```python
from build123d import *

# Parameters (mm, degrees)
SALIENTE_EXTRUIR1_DEPTH = 1.5
CROQUIS2_R              = 1.6
CORTAR_EXTRUIR1_DEPTH   = 3
REDONDEO1_R             = 1
CROQUIS3_R              = 1.5
CORTAR_EXTRUIR2_DEPTH   = 5


with BuildPart() as part:
    # Croquis1 → Saliente-Extruir1 (new, symmetric)
    with BuildSketch(Plane.XY):
        with BuildLine():
            Line((-6, 51), (-6, -10))
            Line((-6, -10), (-3, -10))
            Line((-3, -10), (-3, -55))
            Line((-3, -55), (3, -55))
            Line((3, -55), (3, -10))
            Line((3, -10), (6, -10))
            Line((6, -10), (6, 51))
            ThreePointArc((6, 51), (4.828427125, 53.828427125), (2, 55))
            Line((2, 55), (-2, 55))
            ThreePointArc((-2, 55), (-4.828427125, 53.828427125), (-6, 51))
        make_face()
    extrude(amount=SALIENTE_EXTRUIR1_DEPTH, both=True)

    # Croquis2 → Cortar-Extruir1 (cut)
    with BuildSketch(Plane.XY.offset(1.5)):
        with Locations((0, 50)):
            Circle(CROQUIS2_R)
    extrude(amount=-CORTAR_EXTRUIR1_DEPTH, mode=Mode.SUBTRACT)

    # Redondeo1
    redondeo1_edges = [part.edges().sort_by_distance(p)[0] for p in [
        (3, -55, 0),
        (-3, -55, 0),
    ]]
    fillet(redondeo1_edges, radius=REDONDEO1_R)

    # Croquis3 → Cortar-Extruir2 (cut, symmetric)
    with BuildSketch(Plane.XY):
        Circle(CROQUIS3_R)
    extrude(amount=CORTAR_EXTRUIR2_DEPTH, both=True, mode=Mode.SUBTRACT)


solid = part.part
```
The listing builds one solid part. Answer for the finished solid, in the listing's coordinates (mm). A direction names the side the tool comes from. Round coordinates to 2 decimals unless told otherwise and drop trailing zeros. Order: outer loops, then holes, each group sorted by start corner. A loop starts at its lowest first (then second) coordinate and runs counter-clockwise, first axis right, second up. Notation, with made-up numbers: (82, -3) -> (128, -3) arc R23 cw to (128, 18) -> close; hole circle Ø5 at (6, 24.5). An arc over 180 degrees is marked (long way). Answer as CSV lines item,"result". Start each with the question number.
(1) A tool of negligible diameter and unlimited length cuts with its end or side. For faces 1 (the face through (-6, 21, 0)), 2 (the face through (4, -10, 0)), 3 (the face through (-3, -32, 0)), from which of +Z, -Z, +X, -X, +Y, -Y can it reach the whole face along a straight path? Write none if from no direction.
(2) For a pull along Y with two mould halves and no side action, classify faces 4 (the face through (4.859, 53.797, 0.021)), 5 (the face through (6, 20, 0)), 6 (the face through (-1.5, 0.07, 0.02)) as +Y half, -Y half, draft (parallel to the pull), parting line (faces both ways), or undercut.
(3) Flat-ended cylindrical pins translate along their axes: pin 1 Ø4 at (x, y) = (0, 50) entering from +Z; pin 2 Ø0.9 at (y, z) = (-39.5, -0.5) entering from -X. Find the tip coordinate at first contact, or state that the pin passes through.
(4) The part is cut by section B-B (y = 0). Determine the outline of the cut face in (x, z).
(5) The part is cut by section A-A (x = 0). Determine the outline of the cut face in (y, z).
(6) The part is cut by section D-D (y = -13.5). Determine the outline of the cut face in (x, z), then the cut area to 3 significant figures.
(7) Find the intervals of material crossed by probe 1 along Y at (x, z) = (0, 0.15); probe 2 along Y at (x, z) = (1.25, 0.3); probe 3 along X at (y, z) = (-39, -1), in increasing order. Write a range as from..to.
(8) The part is cut by section C-C (y = 50). Determine the outline of the cut face in (x, z), then the cut area to 3 significant figures.
Evaluation:
1,face 1,"+Z, -Z, -X, +Y, -Y"
1,face 2,"+Z, -Z, +X, -Y"
1,face 3,"+Z, -Z, -X, -Y"
2,face 4,"+Y half"
2,face 5,"draft"
2,face 6,"undercut"
3,pin 1,"z = 1.5"
3,pin 2,"x = -3"
4,outline,"(-6, -1.5) -> (-1.5, -1.5) -> (-1.5, 1.5) -> (-6, 1.5) -> close; (1.5, -1.5) -> (6, -1.5) -> (6, 1.5) -> (1.5, 1.5) -> close"
5,outline,"(-55, -1.5) -> (-1.5, -1.5) -> (-1.5, 1.5) -> (-55, 1.5) -> close; (1.5, -1.5) -> (48.4, -1.5) -> (48.4, 1.5) -> (1.5, 1.5) -> close; (51.6, -1.5) -> (55, -1.5) -> (55, 1.5) -> (51.6, 1.5) -> close"
6,outline,"(-3, -1.5) -> (3, -1.5) -> (3, 1.5) -> (-3, 1.5) -> close"
6,area,"18.0 mm²"
7,probe 1,"-55..-1.5, 1.5..48.4, 51.6..55"
7,probe 2,"-55..-0.83, 0.83..49, 51..55"
7,probe 3,"-3..3"
8,outline,"(-6, -1.5) -> (-1.6, -1.5) -> (-1.6, 1.5) -> (-6, 1.5) -> close; (1.6, -1.5) -> (6, -1.5) -> (6, 1.5) -> (1.6, 1.5) -> close"
8,area,"26.4 mm²"
